Autodesk Inventor part; units mm, degrees
ref_plane "YZ Plane" through (0, 0, 0) normal (1, 0, 0) x (0, 1, 0)
ref_plane "XZ Plane" through (0, 0, 0) normal (0, 1, 0) x (-1, 0, 0)
ref_plane "XY Plane" through (0, 0, 0) normal (0, 0, 1) x (1, 0, 0)
sketch "스케치1" plane through (0, 0, 0) normal (0, 1, 0) x (-1, 0, 0)
  line L0 (-62.3615, 62.3615) -> (-22.8259, 85.1874)
  line L1 (-22.8259, 85.1874) -> (22.8259, 85.1874)
  line L2 (22.8259, 85.1874) -> (62.3615, 62.3615)
  line L3 (62.3615, 62.3615) -> (85.1874, 22.8259)
  line L4 (85.1874, 22.8259) -> (85.1874, -22.8259)
  line L5 (85.1874, -22.8259) -> (62.3615, -62.3615)
  line L6 (62.3615, -62.3615) -> (22.8259, -85.1874)
  line L7 (22.8259, -85.1874) -> (-22.8259, -85.1874)
  line L8 (-22.8259, -85.1874) -> (-62.3615, -62.3615)
  line L9 (-62.3615, -62.3615) -> (-85.1874, -22.8259)
  line L10 (-85.1874, -22.8259) -> (-85.1874, 22.8259)
  line L11 (-85.1874, 22.8259) -> (-62.3615, 62.3615)
  line L12 (88.3874, -23.6833) -> (64.7041, -64.7041)
  line L13 (64.7041, -64.7041) -> (23.6833, -88.3874)
  line L14 (23.6833, -88.3874) -> (-23.6833, -88.3874)
  line L15 (-23.6833, -88.3874) -> (-64.7041, -64.7041)
  line L16 (-64.7041, -64.7041) -> (-88.3874, -23.6833)
  line L17 (-88.3874, -23.6833) -> (-88.3874, 23.6833)
  line L18 (-88.3874, 23.6833) -> (-64.7041, 64.7041)
  line L19 (-64.7041, 64.7041) -> (-23.6833, 88.3874)
  line L20 (-23.6833, 88.3874) -> (23.6833, 88.3874)
  line L21 (23.6833, 88.3874) -> (64.7041, 64.7041)
  line L22 (64.7041, 64.7041) -> (88.3874, 23.6833)
  line L23 (88.3874, 23.6833) -> (88.3874, -23.6833)
  point P0 (0, 0)
  point P1 (0, 0)
  point P2 (0, 0)
  dimension "d0" = 176.385
  dimension "d1" = 3.2
extrude "돌출1" add sketch "스케치1" along normal blind 6.8 contours L0 L1 L2 L3 L4 L5 L6 L7 L8 L9 L10 L11 | L12 L13 L14 L15 L16 L17 L18 L19 L20 L21 L22 L23
sketch "스케치2" plane through (0, 6.8, 0) normal (0, 1, 0) x (1, 0, 0)
  line L0 (-23.2546, 86.7874) -> (23.2546, 86.7874)
  line L1 (23.2546, 86.7874) -> (63.5328, 63.5328)
  line L2 (63.5328, 63.5328) -> (86.7874, 23.2546)
  line L3 (86.7874, 23.2546) -> (86.7874, -23.2546)
  line L4 (86.7874, -23.2546) -> (63.5328, -63.5328)
  line L5 (63.5328, -63.5328) -> (23.2546, -86.7874)
  line L6 (23.2546, -86.7874) -> (-23.2546, -86.7874)
  line L7 (-23.2546, -86.7874) -> (-63.5328, -63.5328)
  line L8 (-63.5328, -63.5328) -> (-86.7874, -23.2546)
  line L9 (-86.7874, -23.2546) -> (-86.7874, 23.2546)
  line L10 (-86.7874, 23.2546) -> (-63.5328, 63.5328)
  line L11 (-63.5328, 63.5328) -> (-23.2546, 86.7874)
  line L12 (-88.3874, 23.6833) -> (-88.3874, -23.6833)
  line L13 (22.7187, -84.7874) -> (-22.7187, -84.7874)
  line L14 (-22.7187, -84.7874) -> (-62.0687, -62.0687)
  line L15 (-62.0687, -62.0687) -> (-84.7874, -22.7187)
  line L16 (-84.7874, -22.7187) -> (-84.7874, 22.7187)
  line L17 (-84.7874, 22.7187) -> (-62.0687, 62.0687)
  line L18 (-62.0687, 62.0687) -> (-22.7187, 84.7874)
  line L19 (-22.7187, 84.7874) -> (22.7187, 84.7874)
  line L20 (22.7187, 84.7874) -> (62.0687, 62.0687)
  line L21 (62.0687, 62.0687) -> (84.7874, 22.7187)
  line L22 (84.7874, 22.7187) -> (84.7874, -22.7187)
  line L23 (84.7874, -22.7187) -> (62.0687, -62.0687)
  line L24 (62.0687, -62.0687) -> (22.7187, -84.7874)
  point P0 (0, 0)
  point P1 (0, 0)
  point P2 (0, 0)
  dimension "d4" = 1.6
  dimension "d5" = 2
extrude "돌출2" cut sketch "스케치2" against normal blind 1.2
sketch "스케치3" plane through (0, 0, 0) normal (0, -1, 0) x (1, 0, 0)
  line L0 (-20, -10) -> (20, -10)
  line L1 (20, -10) -> (20, 10)
  line L2 (20, 10) -> (-20, 10)
  line L3 (-20, 10) -> (-20, -10)
  line L4 (-20, -10) -> (20, 10) construction
  line L5 (20, -10) -> (-20, 10) construction
  point P0 (0, 0)
  point P1 (0, 0)
  point P2 (-20, 0)
  dimension "d8" = 40
  dimension "d9" = 20
extrude "돌출3" add sketch "스케치3" along normal blind 20
sketch "스케치4" plane through (20, 0, -10) normal (0, 0, -1) x (-1, 0, 0)
  circle A0 centre (10, -10) radius 1.25
  line L0 (-3.6833, 0) -> (43.6833, 0)
  line L1 (40, -20) -> (0, -20)
  line L2 (20, -20) -> (20, 0)
  circle A1 centre (20, -10) radius 1.25
  circle A2 centre (30, -10) radius 1.25
  dimension "d13" = 2.5
  dimension "d14" = 10
  dimension "d15" = 10
  dimension "d16" = 2.5
extrude "돌출4" cut sketch "스케치4" against normal blind 20
sketch "스케치5" plane through (0, 6.8, 0) normal (0, 1, 0) x (1, 0, 0)
  line L0 (-62.0687, -62.0687) -> (-22.7187, -84.7874)
  line L1 (-22.7187, -84.7874) -> (22.7187, -84.7874)
  line L2 (22.7187, -84.7874) -> (62.0687, -62.0687)
  line L3 (62.0687, -62.0687) -> (84.7874, -22.7187)
  line L4 (84.7874, -22.7187) -> (84.7874, 22.7187)
  line L5 (84.7874, 22.7187) -> (62.0687, 62.0687)
  line L6 (62.0687, 62.0687) -> (22.7187, 84.7874)
  line L7 (22.7187, 84.7874) -> (-22.7187, 84.7874)
  line L8 (-22.7187, 84.7874) -> (-62.0687, 62.0687)
  line L9 (-62.0687, 62.0687) -> (-84.7874, 22.7187)
  line L10 (-84.7874, 22.7187) -> (-84.7874, -22.7187)
  line L11 (-84.7874, -22.7187) -> (-62.0687, -62.0687)
  point P0 (0, 0)
extrude "돌출5" cut sketch "스케치5" against normal blind 0.6
sketch "스케치6" plane through (0, 0, 0) normal (0, -1, 0) x (1, 0, 0)
  circle A0 centre (0, -52.5) radius 1.25
  line L0 (-20, -10) -> (20, -10)
  point P0 (0, 0)
  point P1 (0, -10)
  dimension "d22" = 2.5
  dimension "d23" = 52.5
extrude "돌출6" cut sketch "스케치6" against normal up to surface (6.2 mm away)
fillet "모깎기1" radius 1.2 24 edges at (76.5457, 0, 44.1937) (76.5457, 6.8, 44.1937) (88.3874, 6.8, 0) (88.3874, 0, 0) (76.5457, 6.8, -44.1937) (76.5457, 0, -44.1937) (44.1937, 6.8, -76.5457) (44.1937, 0, -76.5457) (0, 0, -88.3874) (0, 6.8, -88.3874) (-44.1937, 6.8, -76.5457) (-44.1937, 0, -76.5457) (-76.5457, 0, -44.1937) (-76.5457, 6.8, -44.1937) (-88.3874, 0, 0) (-88.3874, 6.8, 0) (-76.5457, 0, 44.1937) (-76.5457, 6.8, 44.1937) (-44.1937, 0, 76.5457) (-44.1937, 6.8, 76.5457) (0, 0, 88.3874) (0, 6.8, 88.3874) (44.1937, 0, 76.5457) (44.1937, 6.8, 76.5457)
properties part number "(x2)_POSPA_Large_Bottom"
Input: part model. Units: mm. Frame: model coordinates. A direction names the side the tool comes from. Give positions to 0.01 mm unless a question says otherwise; leave off trailing zeros. Order: outer loops, then holes, each group sorted by start corner. A loop starts at its lowest first (then second) coordinate and runs counter-clockwise, first axis right, second up. Notation, with made-up numbers: (87.25, -23) - (105.25, -23) arc R13 cw to (105.25, -8) - close; hole circle Ø2 at (69, 81). An arc over 180 degrees is marked (long way). Answer as a JSON object with one key per item and string values. Group by question number.
Q1. Set-up query: faces 4 (the face through (-44.3, 0.342, 76.067)), 5 (the face through (74.997, 6.208, -43.676)), 6 (the face through (0, -12, -10)). Return all of +Z, -Z, +X, -X, +Y, -Y with unobstructed straight access to the full face (end or side cutting, diameter ignored); none if empty.
Q2. Mould query, pull axis Z, two halves, no side actions, for faces 1 (the face through (-76.067, 0.342, -44.3)), 2 (the face through (-76.38, 3.37, 44.48)), 3 (the face through (-73.587, 5.904, -42.118)). Classes: pulls with the +Z half, pulls with the -Z half, needs draft (parallel to the pull), parting line crosses it, or undercut.
Q3. Line query: probe 1 along Y at (x, z) = (0, -1.25); probe 2 along X at (y, z) = (-11, 9.5); probe 3 along Y at (x, z) = (-20, 13.5). Output: solid intervals per line, ascending.
Q4. Cut plane B-B, the plane z = 20. Output: boundary loops of the cut face in (x, y), then the cut area to 3 significant figures.
Q5. Cut plane A-A, the plane z = 1.5. Output: boundary loops of the cut face in (x, y), then the cut area to 3 significant figures.
Q6. First-contact query: pin 1 Ø10 at (y, z) = (-8, -4.5) entering from -X; pin 2 Ø3 at (x, z) = (0, -52.5) entering from -Y; pin 3 Ø16 at (x, y) = (2.5, -12.5) entering from -Z. Flat tips, straight axial feed; report the tip coordinate or a pass-through.
Q7. Cut plane C-C, the plane y = -15.5. Output: boundary loops of the cut face in (x, z), then the cut area to 3 significant figures.
Results:
{
 "1": {"face 4": "+Z, -X, -Y", "face 5": "+Y", "face 6": "-Z, +X, -X, -Y"},
 "2": {"face 1": "pulls with the -Z half", "face 2": "pulls with the +Z half", "face 3": "undercut"},
 "3": {"probe 1": "-20 to -11.25, -8.75 to 6.2", "probe 2": "-20 to -10.75, -9.25 to -0.75, 0.75 to 9.25, 10.75 to 20", "probe 3": "0 to 6.2"},
 "4": {"outline": "(-88.39, 1.2) arc R1.2 ccw to (-87.19, 0) - (87.19, 0) arc R1.2 ccw to (88.39, 1.2) - (88.39, 5.6) arc R1.2 ccw to (87.19, 6.8) - (86.79, 6.8) - (86.79, 5.6) - (84.79, 5.6) - (84.79, 6.2) - (-84.79, 6.2) - (-84.79, 5.6) - (-86.79, 5.6) - (-86.79, 6.8) - (-87.19, 6.8) arc R1.2 ccw to (-88.39, 5.6) - close", "area": "1,090 mm^2"},
 "5": {"outline": "(-88.39, 1.2) arc R1.2 ccw to (-87.19, 0) - (-20, 0) - (-20, -20) - (20, -20) - (20, 0) - (87.19, 0) arc R1.2 ccw to (88.39, 1.2) - (88.39, 5.6) arc R1.2 ccw to (87.19, 6.8) - (86.79, 6.8) - (86.79, 5.6) - (84.79, 5.6) - (84.79, 6.2) - (-84.79, 6.2) - (-84.79, 5.6) - (-86.79, 5.6) - (-86.79, 6.8) - (-87.19, 6.8) arc R1.2 ccw to (-88.39, 5.6) - close; hole circle Ø2.5 at (-10, -10); hole circle Ø2.5 at (0, -10); hole circle Ø2.5 at (10, -10)", "area": "1,880 mm^2"},
 "6": {"pin 1": "x = -20", "pin 2": "y = 0", "pin 3": "z = -10"},
 "7": {"outline": "(-20, -10) - (20, -10) - (20, 10) - (-20, 10) - close", "area": "800 mm^2"}
}
